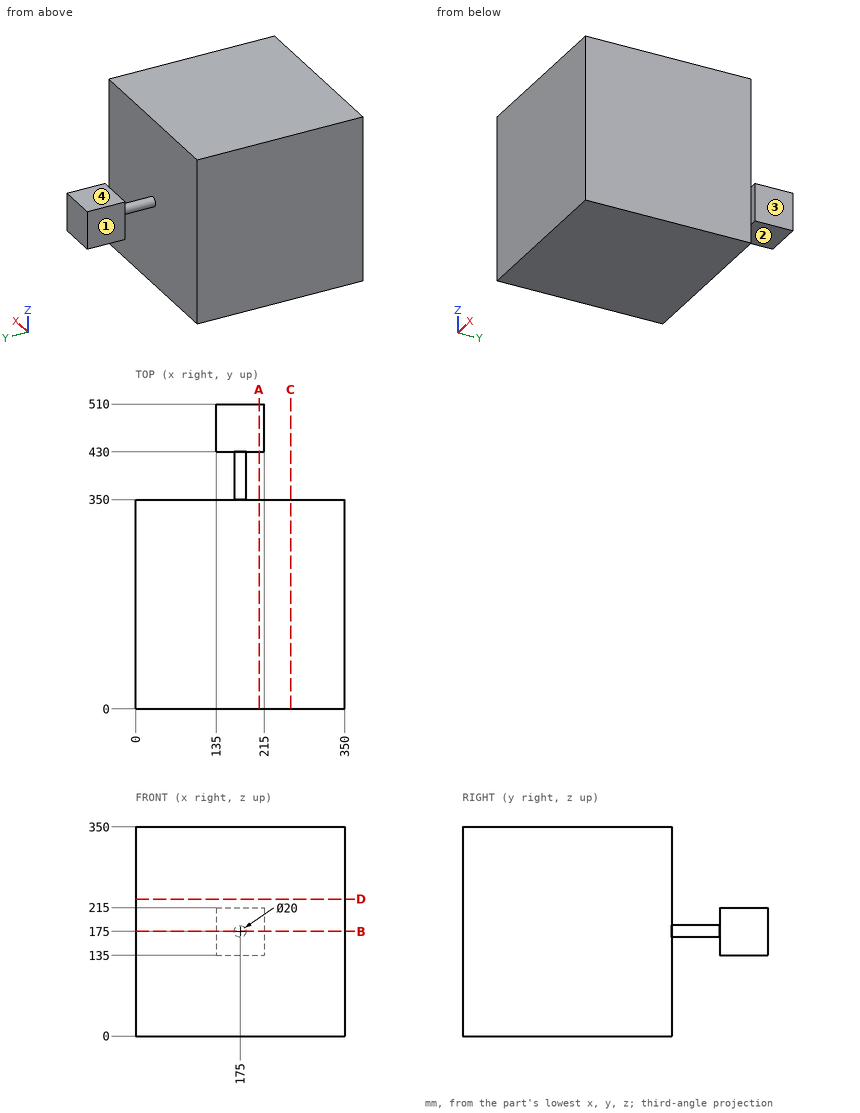
The figure shows three views and two pictorial views of one solid part (mm, origin at its lowest corner). Answer the questions. A direction names the side the tool comes from. Give positions to 0.01 mm unless a question says otherwise; leave off trailing zeros. Order: outer loops, then holes, each group sorted by start corner. A loop starts at its lowest first (then second) coordinate and runs counter-clockwise, first axis right, second up. Notation, with made-up numbers: (19.5, 69) -> (65.5, 69) arc R23 cw to (65.5, 104) -> close; hole circle Ø1 at (16.25, -19). An arc over 180 degrees is marked (long way). Answer as a JSON object with one key per item and string values. Group by question number.
Item 1: A tool of negligible diameter and unlimited length cuts with its end or side. For the marked faces 1, 2, 3 and 4, from which of +Z, -Z, +X, -X, +Y, -Y can it reach the whole face along a straight path? Write none if from no direction.
Item 2: The part is cut by section C-C on x = 259.5. Write down the section's boundary in (y, z).
Item 3: Consider L1, parallel to Y at x = 32, z = 142.5. Determine where the line is inside the solid, lowest interval first. Write a range as from..to.
Item 4: The part is cut by section B-B on z = 175. Write down the section's boundary in (x, y).
Item 5: The part is cut by section A-A on x = 207. Write down the section's boundary in (y, z).
Item 6: Flat-ended cylindrical pins translate along their axes: pin 1 (8 mm diameter, centred on x = 60.5, z = 142.5, fed in from +Y); pin 2 (6 mm diameter, centred on x = 177.5, y = 369, fed in from -Z); pin 3 (24 mm diameter, centred on y = 473, z = 191.5, fed in from -X). Find the tip coordinate at first contact, or state that the pin passes through.
Result set:
{
 "1": {"face 1": "+Z, -Z, -X, +Y", "face 2": "-Z, +X, -X, +Y", "face 3": "+Z, -Z, +X, +Y", "face 4": "+Z, +X, -X, +Y"},
 "2": {"outline": "(0, 0) -> (350, 0) -> (350, 350) -> (0, 350) -> close"},
 "3": {"L1": "0..350"},
 "4": {"outline": "(0, 0) -> (350, 0) -> (350, 350) -> (185, 350) -> (185, 430) -> (215, 430) -> (215, 510) -> (135, 510) -> (135, 430) -> (165, 430) -> (165, 350) -> (0, 350) -> close"},
 "5": {"outline": "(0, 0) -> (350, 0) -> (350, 350) -> (0, 350) -> close; (430, 135) -> (510, 135) -> (510, 215) -> (430, 215) -> close"},
 "6": {"pin 1": "y = 350", "pin 2": "z = 165", "pin 3": "x = 135"}
}
